Input: part model. Units: mm. Frame: model coordinates. Coordinates: 2 decimals unless noted, no trailing zeros. Write each loop counter-clockwise with the first axis right and the second up, starting at its lowest first coordinate (ties: lowest second). Pieces come first, ordered by that corner, then holes. Notation, with made-up numbers: M 32,10.25 L 61,10.25 A16 cw 61,28.25 Z; hole C 44.25,76.5 d9. An arc over 180 degrees is marked long. Use one line per item in the form item = value.
Autodesk Inventor part; units mm, degrees
ref_plane "YZ Plane" through (0, 0, 0) normal (1, 0, 0) x (0, 1, 0)
ref_plane "XZ Plane" through (0, 0, 0) normal (0, 1, 0) x (-1, 0, 0)
ref_plane "XY Plane" through (0, 0, 0) normal (0, 0, 1) x (1, 0, 0)
sketch "Sketch1" plane through (0, 0, 0) normal (0, 0, 1) x (1, 0, 0)
  line L0 (-7.5883, 0) -> (7.5883, 0)
  line L1 (7.5883, 0) -> (7.5883, 1.3208)
  line L2 (7.5883, 1.3208) -> (6.8262, 2.0828)
  line L3 (6.8262, 2.0828) -> (-2.7622, 2.0828)
  line L4 (-2.7622, 2.0828) -> (-3.5242, 1.3208)
  line L5 (-3.5242, 1.3208) -> (-3.5242, 0.889)
  line L6 (-3.5242, 0.889) -> (-6.6993, 0.889)
  arc A0 (-6.6993, 0.889) -> (-7.5883, 0) centre (-6.6993, 0) ccw
  point P0 (0, 0)
  point P1 (0, 0)
  dimension "d0" = 4.1656
  dimension "d1" = 11.1125
  dimension "d2" = 1.778
  dimension "d3" = 0.762
  dimension "d4" = 4.064
revolve "Revolution1" add sketch "Sketch1" angle 360 about axis through (-7.5883, 0, 0) along (1, 0, 0)
sketch "Sketch2" plane through (7.5883, 0, 0) normal (1, 0, 0) x (0, 0, -1)
  circle A0 centre (0, 0) radius 2.0828
  circle A1 centre (0, 0) radius 1.3208
  line L0 (-2.0828, 0.508) -> (2.0828, 0.508)
  line L1 (2.0828, 0.508) -> (2.0828, -0.508)
  line L2 (2.0828, -0.508) -> (-2.0828, -0.508)
  line L3 (-2.0828, -0.508) -> (-2.0828, 0.508)
  point P0 (0, 0)
  point P1 (-2.0828, 0)
  dimension "d6" = 1.016
extrude "Extrusion1" cut sketch "Sketch2" against normal blind 0.762 contours A0 L2 A1 L0 | L1 L2 A0 | A0 L0 L1 | L0 A1 L2 A0 | A0 L3 L0 | A1 L2 L0 | L2 L3 A0
thread "Thread1"
sketch "Sketch3" plane through (-3.5242, 0, 0) normal (-1, 0, 0) x (0, 0, 1)
  arc A0 (2.0199, -0.508) -> (2.0199, 0.508) centre (0, 0) ccw
  line L0 (-2.0199, -0.508) -> (2.0199, -0.508)
  arc A1 (-2.0199, 0.508) -> (-2.0199, -0.508) centre (0, 0) ccw
  line L1 (2.0199, 0.508) -> (-2.0199, 0.508)
  circle A2 centre (0, 0) radius 0.889
  circle A3 centre (0, 0) radius 1.3208
  arc A4 (-0.7296, 0.508) -> (-0.7296, -0.508) centre (0, 0) ccw
  arc A5 (0.7296, -0.508) -> (0.7296, 0.508) centre (0, 0) ccw
  point P0 (0, 0)
extrude "Extrusion2" cut sketch "Sketch3" against normal blind 0.762 contours L0 A3 L1 A0 | L0 A2 L1 A3 | A3 L1 A2 L0 | L0 A1 L1 A3
properties part number "Spring_Separation" material "Stainless Steel"
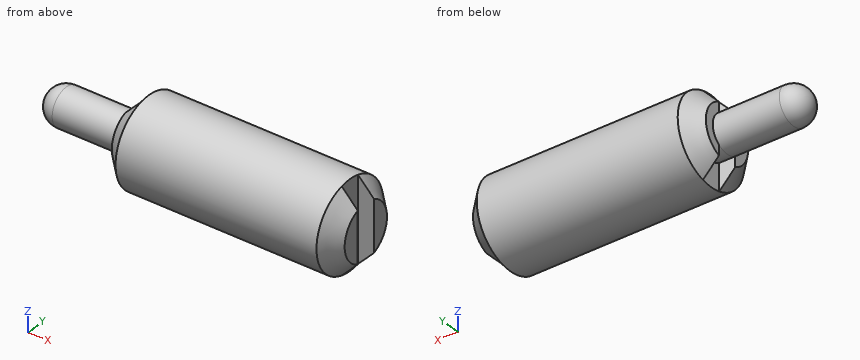
(1) Section query C-C on x = -5.75. Return the cut outline in (y, z), plus the area to 3 significant figures.
Computed:
outline = C 0,0 d1.78
area = 2.48 mm^2
(2) Section query A-A on z = 0. Return the cut outline in (x, y), plus the area to 3 significant figures.
Computed:
outline = M -6.7,-0.89 L -3.52,-0.89 L -3.52,-1.32 L -2.76,-2.08 L 6.83,-2.08 L 7.59,-1.32 L 7.59,-0.51 L 6.83,-0.51 L 6.83,0.51 L 7.59,0.51 L 7.59,1.32 L 6.83,2.08 L -2.76,2.08 L -3.52,1.32 L -3.52,0.89 L -6.7,0.89 A0.89 ccw Z
area = 51.2 mm^2
(3) Line query: probe 1 along X at (y, z) = (-0.2, 1.15); probe 2 along X at (y, z) = (-0.65, -1); probe 3 along Z at (x, y) = (1.75, 0.1). Output: solid intervals per line, ascending.
Computed:
probe_1 = -2.76 to 6.83
probe_2 = -3.52 to 7.59
probe_3 = -2.08 to 2.08
(4) First-contact query: pin 1 Ø0.5 at (y, z) = (0, 1.5) entering from -X; pin 2 Ø0.6 at (x, z) = (-3, 1) entering from +Y; pin 3 Ø0.8 at (x, z) = (7, -0.5) entering from -Y. Flat tips, straight axial feed; report the tip coordinate or a pass-through.
Computed:
pin_1 = -2.76
pin_2 = 1.92
pin_3 = -2.08
(5) Section query D-D on x = 2. Return the cut outline in (y, z).
Computed:
outline = C 0,0 d4.17
